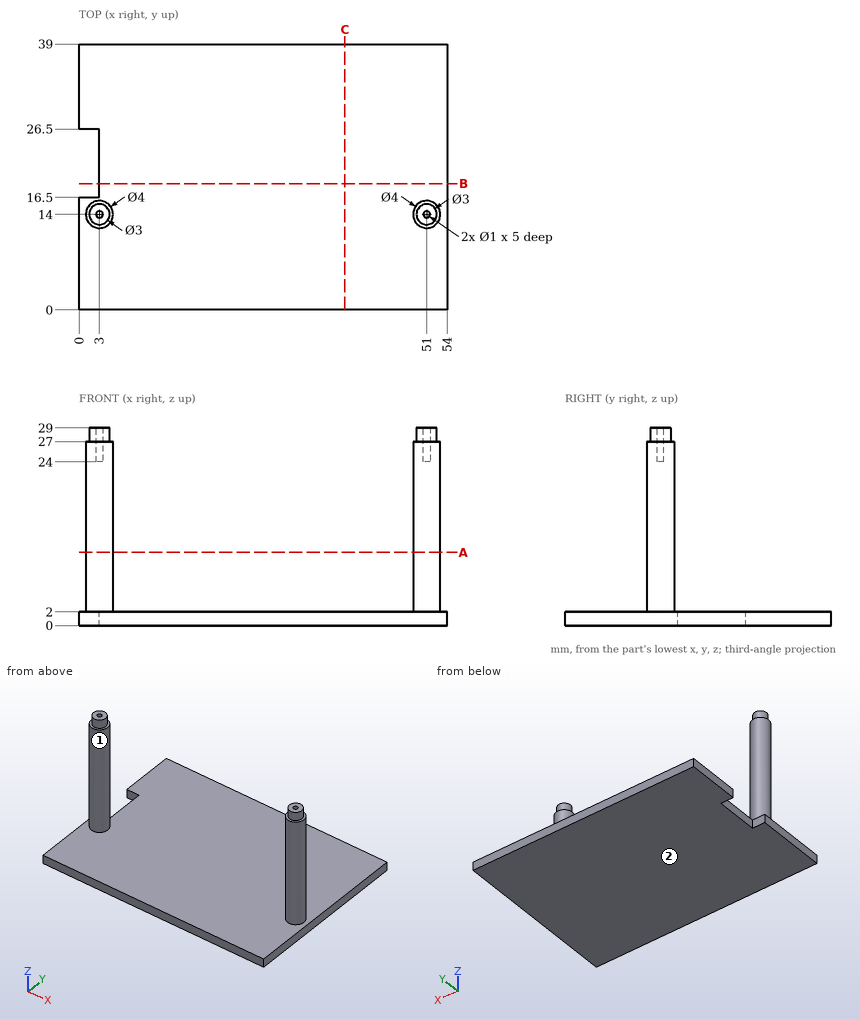
Design review of the part shown in the three views and the two pictorial views. Dimensions are in mm from the part's minimum x, y and z. Round coordinates to 2 decimals unless told otherwise and drop trailing zeros. Order: outer loops, then holes, each group sorted by start corner. A loop starts at its lowest first (then second) coordinate and runs counter-clockwise, first axis right, second up. Notation, with made-up numbers: (1.5, -39.5) -> (27.5, -39.5) arc R8 cw to (27.5, -24.5) -> close; hole circle Ø11 at (57.5, -6.75). An arc over 180 degrees is marked (long way). Write item = value, one per line. Start each with the question number.
1) To check wall thickness, follow line 1 (Y direction, x = 51, z = 27.6); line 2 (Y direction, x = 51, z = 26.15); line 3 (Z direction, x = 3.5, y = 27). State the ranges of each line that lie inside material, in increasing order. Write a range as from..to.
2) Take a section at B-B on y = 18.5. State the section outline as (x, z) points.
3) Insertion check: pin 1 (4 mm diameter, centred on y = 14, z = 11, fed in from -X); pin 2 (11.5 mm diameter, centred on x = 32, y = 18, fed in from +Z); pin 3 (0.5 mm diameter, centred on x = 3, y = 14, fed in from +Z); pin 4 (8 mm diameter, centred on y = 21.5, z = 9.5, fed in from +X). Each pin has a flat end and moves straight along its axis. Give the tip position at first contact, or say it passes through.
4) The part is to be moulded in two halves that separate along X. For the marked faces 1 and 2, say which applies: +X half, -X half, draft (parallel to the pull), parting line (faces both ways), or undercut.
5) Take a section at A-A on z = 10.75. State the section outline as (x, y) points.
6) Take a section at C-C on x = 39. State the section outline as (y, z) points.
Verdict:
q1.line_1 = 12.5..13.5, 14.5..15.5
q1.line_2 = 12..13.5, 14.5..16
q1.line_3 = 0..2
q2.outline = (3, 0) -> (54, 0) -> (54, 2) -> (3, 2) -> close
q3.pin_1 = 1
q3.pin_2 = 2
q3.pin_3 = 24
q3.pin_4 = through
q4.face_1 = undercut
q4.face_2 = draft
q5.outline = circle Ø4 at (3, 14); circle Ø4 at (51, 14)
q6.outline = (0, 0) -> (39, 0) -> (39, 2) -> (0, 2) -> close
